Check sheet for the modelled part. Datum: model origin and axes. Units: mm. A direction names the side the tool comes from. Give positions to 0.01 mm unless a question says otherwise; leave off trailing zeros. Order: outer loops, then holes, each group sorted by start corner. A loop starts at its lowest first (then second) coordinate and runs counter-clockwise, first axis right, second up. Notation, with made-up numbers: (-34.75, 36.25) -> (-2.75, 36.25) arc R13 ccw to (-2.75, 57.25) -> close; hole circle Ø3 at (89, 74). An arc over 180 degrees is marked (long way). Answer in a Markdown table with one row per item. Add a question column.
(1) Cross-section at A-A (x = 0). Record the cut outline in (y, z), then the cut area to 3 significant figures.
(2) Cross-section at C-C (y = 16.5). Record the cut outline in (x, z), then the cut area to 3 significant figures.
(3) Set-up check for faces 1 (the face through (0.45, 12.41, 1.43)), 2 (the face through (0.45, 2.76, 1.43)), 3 (the face through (0, 0, 0)): record each of +Z, -Z, +X, -X, +Y, -Y from which the full face is reachable in a straight line by a thin tool's end or side.
(4) Thickness scan on L1, parallel to Y at x = -1.45, z = 0.7; L2, parallel to X at y = 14, z = 0.1; L3, parallel to X at y = 16.75, z = -1.3. Record the ranges inside material, lowest first. Write a range as [from, to].
(5) Cross-section at B-B (z = 0). Record the cut outline in (x, y), then the cut area to 3 significant figures.
(6) Go/stop test with flat-tipped pins: pin 1 (3 mm diameter, centred on y = 10, z = 0, fed in from -X); pin 2 (2 mm diameter, centred on y = 3.5, z = -1, fed in from +X); pin 3 (3 mm diameter, centred on x = 1, y = 2, fed in from -Z). Record where each tip stops, or that it passes through.
```python
from build123d import *

# Parameters (mm, degrees)
SKETCH_1_R      = 1.5
EXTRUDE_1_DEPTH = 19
EXTRUDE_START   = -5.5
SKETCH_3_R      = 2.5
SKETCH_3_R_2    = 1.5
EXTRUDE_3_DEPTH = 0.5
FILLET_1_R      = 0.1


with BuildPart() as part:
    # 草图1 → 凸台-拉伸1 (new body)
    with BuildSketch(Plane(origin=(0, 0, 0), x_dir=(1, 0, 0), z_dir=(0, 1, 0))):
        with Locations(Location((0, 0, 0), (0, 0, 270))):
            Circle(SKETCH_1_R)
    extrude(amount=EXTRUDE_1_DEPTH)

    # 草图3 → 凸台-拉伸3 (add)
    with BuildSketch(Plane(origin=(0, 0, 0), x_dir=(-1, 0, 0), z_dir=(0, -1, 0)).offset(EXTRUDE_START)):
        with Locations(Location((0, 0, 0), (0, 0, 90))):
            Circle(SKETCH_3_R)
        with Locations(Location((0, 0, 0), (0, 0, 90))):
            Circle(SKETCH_3_R_2, mode=Mode.SUBTRACT)
    extrude(amount=-EXTRUDE_3_DEPTH)

    # 圆角1
    fillet_1_edges = [part.edges().sort_by_distance(p)[0] for p in [
        (0, 0, -1.5),
        (0, 19, -1.5),
        (0, 6, -1.5),
        (0, 5.5, 2.5),
        (0, 6, 2.5),
    ]]
    fillet(fillet_1_edges, radius=FILLET_1_R)


solid = part.part
```
Answer below:
| question | item | result |
|---|---|---|
| 1 | outline | (0, -1.4) arc R0.1 ccw to (0.1, -1.5) -> (5.5, -1.5) -> (5.5, -2.4) arc R0.1 ccw to (5.6, -2.5) -> (5.9, -2.5) arc R0.1 ccw to (6, -2.4) -> (6, -1.6) arc R0.1 cw to (6.1, -1.5) -> (18.9, -1.5) arc R0.1 ccw to (19, -1.4) -> (19, 1.4) arc R0.1 ccw to (18.9, 1.5) -> (6.1, 1.5) arc R0.1 cw to (6, 1.6) -> (6, 2.4) arc R0.1 ccw to (5.9, 2.5) -> (5.6, 2.5) arc R0.1 ccw to (5.5, 2.4) -> (5.5, 1.5) -> (0.1, 1.5) arc R0.1 ccw to (0, 1.4) -> close |
| 1 | area | 58.0 mm² |
| 2 | outline | circle Ø3 at (0, 0) |
| 2 | area | 7.07 mm² |
| 3 | face 1 | +Y |
| 3 | face 2 | -Y |
| 3 | face 3 | +Z, -Z, +X, -X, -Y |
| 4 | L1 | y = [5.5, 6] |
| 4 | L2 | x = [-1.5, 1.5] |
| 4 | L3 | x = [-0.75, 0.75] |
| 5 | outline | (-2.5, 5.6) arc R0.1 ccw to (-2.4, 5.5) -> (-1.5, 5.5) -> (-1.5, 0.1) arc R0.1 ccw to (-1.4, 0) -> (1.4, 0) arc R0.1 ccw to (1.5, 0.1) -> (1.5, 5.5) -> (2.4, 5.5) arc R0.1 ccw to (2.5, 5.6) -> (2.5, 5.9) arc R0.1 ccw to (2.4, 6) -> (1.6, 6) arc R0.1 cw to (1.5, 6.1) -> (1.5, 18.9) arc R0.1 ccw to (1.4, 19) -> (-1.4, 19) arc R0.1 ccw to (-1.5, 18.9) -> (-1.5, 6.1) arc R0.1 cw to (-1.6, 6) -> (-2.4, 6) arc R0.1 ccw to (-2.5, 5.9) -> close |
| 5 | area | 58.0 mm² |
| 6 | pin 1 | stops at x = -1.5 |
| 6 | pin 2 | stops at x = 1.5 |
| 6 | pin 3 | stops at z = -1.5 |
